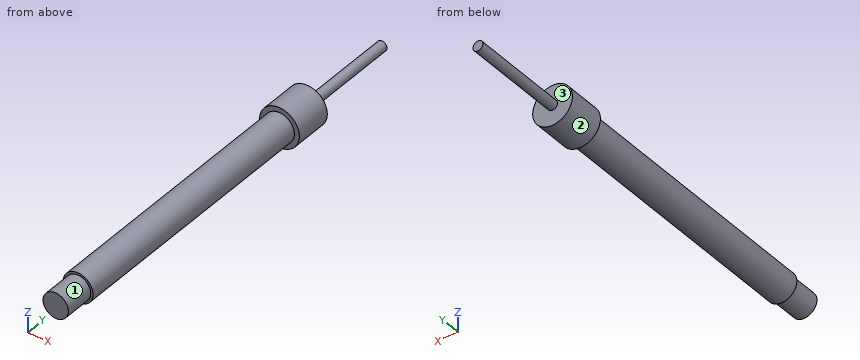
```python
from build123d import *

# Parameters (mm, degrees)
SKETCH1_R       = 5.1
GLASS_TIP_DEPTH = 12
BODY_START      = 12
SKETCH2_R       = 6
BODY_DEPTH      = 108
CAP_START       = 120
SKETCH3_R       = 8
CAP_DEPTH       = 15
CABLE_START     = 135
SKETCH4_R       = 2
CABLE_DEPTH     = 40


with BuildPart() as part:
    # Sketch1 → Glass_Tip (new body)
    with BuildSketch(Plane(origin=(0, 0, 0), x_dir=(1, 0, 0), z_dir=(0, 1, 0))):
        with Locations(Location((0, 0, 0), (0, 0, 270))):
            Circle(SKETCH1_R)
    extrude(amount=GLASS_TIP_DEPTH)

    # Sketch2 → Body (add)
    with BuildSketch(Plane(origin=(0, 0, 0), x_dir=(1, 0, 0), z_dir=(0, 1, 0)).offset(BODY_START)):
        with Locations(Location((0, 0, 0), (0, 0, 270))):
            Circle(SKETCH2_R)
    extrude(amount=BODY_DEPTH)

    # Sketch3 → Cap (add)
    with BuildSketch(Plane(origin=(0, 0, 0), x_dir=(1, 0, 0), z_dir=(0, 1, 0)).offset(CAP_START)):
        with Locations(Location((0, 0, 0), (0, 0, 270))):
            Circle(SKETCH3_R)
    extrude(amount=CAP_DEPTH)

    # Sketch4 → Cable (add)
    with BuildSketch(Plane(origin=(0, 0, 0), x_dir=(1, 0, 0), z_dir=(0, 1, 0)).offset(CABLE_START)):
        with Locations(Location((0, 0, 0), (0, 0, 270))):
            Circle(SKETCH4_R)
    extrude(amount=CABLE_DEPTH)


solid = part.part
```
The listing builds one solid part. Answer for the finished solid, in the listing's coordinates (mm). Face numbers are marked on the shaded views. A direction names the side the tool comes from. Coordinates: 2 decimals unless noted, no trailing zeros. Write each loop counter-clockwise with the first axis right and the second up, starting at its lowest first coordinate (ties: lowest second). Pieces come first, ordered by that corner, then holes.
Q1. Find the intervals of material crossed by line 1 along Y through (x, z) = (-3.5, -3.75); line 2 along Y through (x, z) = (2, 2); line 3 along X through (y, z) = (69.5, 2.25), in increasing order.
Returned:
line 1: y = 12 to 135
line 2: y = 0 to 135
line 3: x = -5.56 to 5.56
Q2. Given P1, Ø2, axis at x = 3, z = 3, coming from the -Y side; P2, Ø6, axis at y = 118, z = -5, coming from the -X side; P3, Ø3, axis at y = 115, z = 5.5, coming from the +X side; P4, Ø1.5, axis at y = 60, z = -5.5, coming from the -X side, each flat-ended and moving along its own axis, determine where each tip first touches the part or whether it passes through.
Returned:
P1: stops at y = 0
P2: stops at x = -7.51
P3: stops at x = 4.47
P4: stops at x = -3.67
Q3. Section A-A, the plane z = 0 is taken. Write down the section's boundary in (x, y), then the cut area to 3 significant figures.
Returned:
outline: (-8, 120) - (-6, 120) - (-6, 12) - (-5.1, 12) - (-5.1, 0) - (5.1, 0) - (5.1, 12) - (6, 12) - (6, 120) - (8, 120) - (8, 135) - (2, 135) - (2, 175) - (-2, 175) - (-2, 135) - (-8, 135) - close
area: 1,820 mm2
Q4. Which of the six approach directions +Z, -Z, +X, -X, +Y, -Y give full straight-line access (tool end or side, diameter ignored) to the marked faces 1, 2 and 3?
Returned:
face 1: -Y
face 2: +Y, -Y
face 3: +Y
Q5. Section C-C, the plane y = 30 is taken. Write down the section's boundary in (x, z), then the cut area to 3 significant figures.
Returned:
outline: circle Ø12 at (0, 0)
area: 113 mm2
Q6. Section B-B, the plane x = 0 is taken. Write down the section's boundary in (y, z), then the cut area to 3 significant figures.
Returned:
outline: (0, -5.1) - (12, -5.1) - (12, -6) - (120, -6) - (120, -8) - (135, -8) - (135, -2) - (175, -2) - (175, 2) - (135, 2) - (135, 8) - (120, 8) - (120, 6) - (12, 6) - (12, 5.1) - (0, 5.1) - close
area: 1,820 mm2
Q7. Section D-D, the plane y = 126.5 is taken. Write down the section's boundary in (x, z).
Returned:
outline: circle Ø16 at (0, 0)
